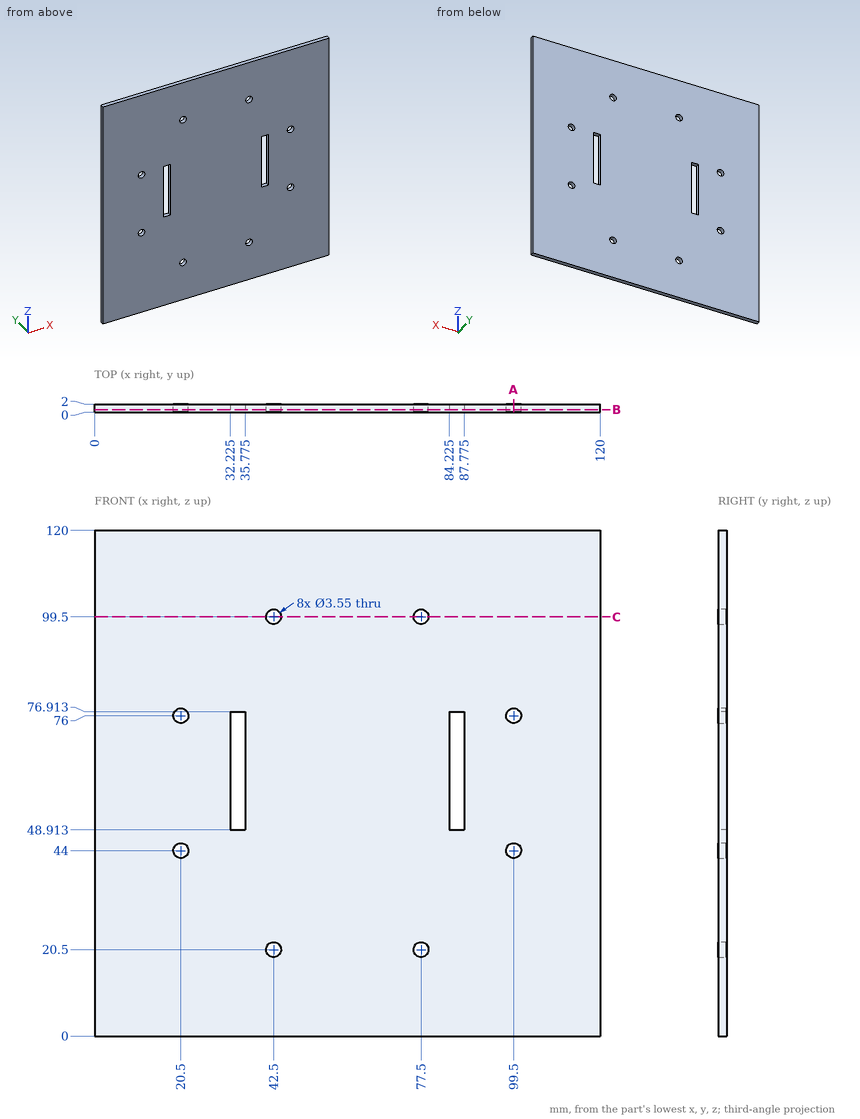
Geometry check sheet. Reference: drawing and pictorial views, mm from the part's lowest x, y, z. Coordinates: 2 decimals unless noted, no trailing zeros. Write each loop counter-clockwise with the first axis right and the second up, starting at its lowest first coordinate (ties: lowest second). Pieces come first, ordered by that corner, then holes. Notation, with made-up numbers: (29, 47) -> (78, 47) arc R12 cw to (78, 57) -> close; hole circle Ø4 at (58, -7.75). An arc over 180 degrees is marked (long way). One line per question, with ' | ' between items.
1. Thickness scan on probe 1 along X at (y, z) = (1.1, 44) (1 decimal); probe 2 along X at (y, z) = (0.75, 76) (1 decimal); probe 3 along X at (y, z) = (0.6, 20.5) (1 decimal). Record the ranges inside material, lowest first. Write a range as from..to.
Answers:
probe 1: x = 0..18.7, 22.3..97.7, 101.3..120 | probe 2: x = 0..18.7, 22.3..32.2, 35.8..84.2, 87.8..97.7, 101.3..120 | probe 3: x = 0..40.7, 44.3..75.7, 79.3..120
2. Cross-section at B-B on y = 0.65. State how many separate pieces and enclosed holes the cut face has, and give its area (3 significant figures).
Answers:
separate pieces: 1 | enclosed holes: 10 | area: 14,100 mm²
3. Cross-section at C-C on z = 99.5. Record the cut outline in (x, y) (1 decimal).
Answers:
outline: (0, 0) -> (40.7, 0) -> (40.7, 2) -> (0, 2) -> close; (44.3, 0) -> (75.7, 0) -> (75.7, 2) -> (44.3, 2) -> close; (79.3, 0) -> (120, 0) -> (120, 2) -> (79.3, 2) -> close
4. Cross-section at A-A on x = 99.5. Record the cut outline in (y, z) (1 decimal), and give its area (3 significant figures).
Answers:
outline: (0, 0) -> (2, 0) -> (2, 42.2) -> (0, 42.2) -> close; (0, 45.8) -> (2, 45.8) -> (2, 74.2) -> (0, 74.2) -> close; (0, 77.8) -> (2, 77.8) -> (2, 120) -> (0, 120) -> close | area: 226 mm²
